```python
from build123d import *

# Parameters (mm, degrees)
F0_W     = 38.1
F0_H     = 31.75
F1_DEPTH = 25.4
F4_DEPTH = 25.4
F5_DEPTH = 12.7


with BuildPart() as f1:
    # F0 (on Front) → F1 (new body)
    with BuildSketch(Plane.XZ):
        with Locations((19.05, 15.875)):
            Rectangle(F0_W, F0_H)
    extrude(amount=F1_DEPTH)

    # F3 (on face) → F4 (cut)
    with BuildSketch(Plane.XY.offset(31.75)):
        Polygon((37.9892475903, 0), (37.9892475903, -12.7), (25.3008189245, -12.1579870905), (25.3008189245, 0), (12.7, 0), (12.7, -12.7), (0, -12.7), (0, -25.4), (38.1, -25.4), (38.1, 0), align=None)
    extrude(amount=-F4_DEPTH, mode=Mode.SUBTRACT)

    # F5 (add): a face of the model
    f5_faces = [f1.faces().sort_by_distance(p)[0] for p in [
        (19.1345000359, -15.8550557875, 6.35),
    ]]
    extrude(f5_faces, amount=F5_DEPTH)


solid = f1.part
```
The listing builds one solid part. Answer for the finished solid, in the listing's coordinates (mm). A direction names the side the tool comes from. Give positions to 0.01 mm unless a question says otherwise; leave off trailing zeros. Order: outer loops, then holes, each group sorted by start corner. A loop starts at its lowest first (then second) coordinate and runs counter-clockwise, first axis right, second up. Notation, with made-up numbers: (3, 14.25) - (12, 14.25) arc R21 ccw to (12, 33.25) - close; hole circle Ø6 at (-6, 78). An arc over 180 degrees is marked (long way). Use one line per item in the form item = value. Start each with the question number.
(1) A cutting plane is placed at A-A, the plane z = 28. Write down the section's boundary in (x, y), then the cut area to 3 significant figures.
(2) The mould has two halves that part along X. Classify faces 1 (the flat face through (19, -15, 19.05)), 2 (the flat face through (0, -10, 12)), 3 (the flat face through (32, -6, 31.75)), 4 (the flat face through (12.7, -6, 25)): released by +X, released by -X, zero draft, split by the parting line, or undercut.
(3) For faces 5 (the flat face through (37.989, -6, 25)), 6 (the flat face through (31.734, -12.433, 25.489)), 7 (the flat face through (25.301, -6, 25)), 8 (the flat face through (6, -12.7, 25)), determine the directions among +Z, -Z, +X, -X, +Y, -Y from which every point of the face is accessible in a straight line to the end or side of a thin tool.
(4) A cutting plane is placed at D-D, the plane x = 27.5. Write down the section's boundary in (y, z).
(5) Consider line 1 (Z direction, x = 13, y = -19.75); line 2 (Y direction, x = 4, z = 27); line 3 (Y direction, x = 28, z = 25). Determine where each line is inside the solid, lowest interval first. Write a range as from..to.
(6) Flat-ended cylindrical pins translate along their axes: pin 1 Ø1.5 at (x, y) = (24, -16.5) entering from +Z; pin 2 Ø10 at (y, z) = (-5.5, 27.5) entering from +X; pin 3 Ø4 at (x, z) = (7.5, 24) entering from -Y. Find the tip coordinate at first contact, or state that the pin passes through.
(7) A cutting plane is placed at B-B, the plane y = -2.5. Write down the section's boundary in (x, z), then the cut area to 3 significant figures.
(8) A cutting plane is placed at C-C, the plane x = 2. Write down the section's boundary in (y, z), then the cut area to 3 significant figures.
Ans:
q1.outline = (0, -12.7) - (12.7, -12.7) - (12.7, 0) - (0, 0) - close; (25.3, -12.16) - (37.99, -12.7) - (37.99, 0) - (25.3, 0) - close
q1.area = 319 mm^2
q2.face_1 = undercut
q2.face_2 = released by -X
q2.face_3 = zero draft
q2.face_4 = undercut
q3.face_5 = +Z, +X, +Y, -Y
q3.face_6 = +Z, -Y
q3.face_7 = +Z, +Y, -Y
q3.face_8 = +Z, +X, -X, -Y
q4.outline = (-25.4, 0) - (0, 0) - (0, 31.75) - (-12.25, 31.75) - (-12.25, 19.05) - (-25.4, 19.05) - close
q5.line_1 = 0..19.05
q5.line_2 = -12.7..0
q5.line_3 = -12.27..0
q6.pin_1 = 19.05
q6.pin_2 = 37.99
q6.pin_3 = -12.7
q7.outline = (0, 0) - (38.1, 0) - (38.1, 19.05) - (37.99, 19.05) - (37.99, 31.75) - (25.3, 31.75) - (25.3, 19.05) - (12.7, 19.05) - (12.7, 31.75) - (0, 31.75) - close
q7.area = 1,050 mm^2
q8.outline = (-25.4, 0) - (0, 0) - (0, 31.75) - (-12.7, 31.75) - (-12.7, 19.05) - (-25.4, 19.05) - close
q8.area = 645 mm^2
